Can you work these out from the drawing? Everything is in mm from the part's minimum corner. A direction names the side the tool comes from. Coordinates: 2 decimals unless noted, no trailing zeros. Order: outer loops, then holes, each group sorted by start corner. A loop starts at its lowest first (then second) coordinate and runs counter-clockwise, first axis right, second up. Notation, with made-up numbers: (82.25, 18) - (108.25, 18) arc R27 ccw to (108.25, 43) - close; hole circle Ø3 at (37, -8.5). An arc over 180 degrees is marked (long way). Use CSV: the item, a comma, the result in double quotes. Start each with the question number.
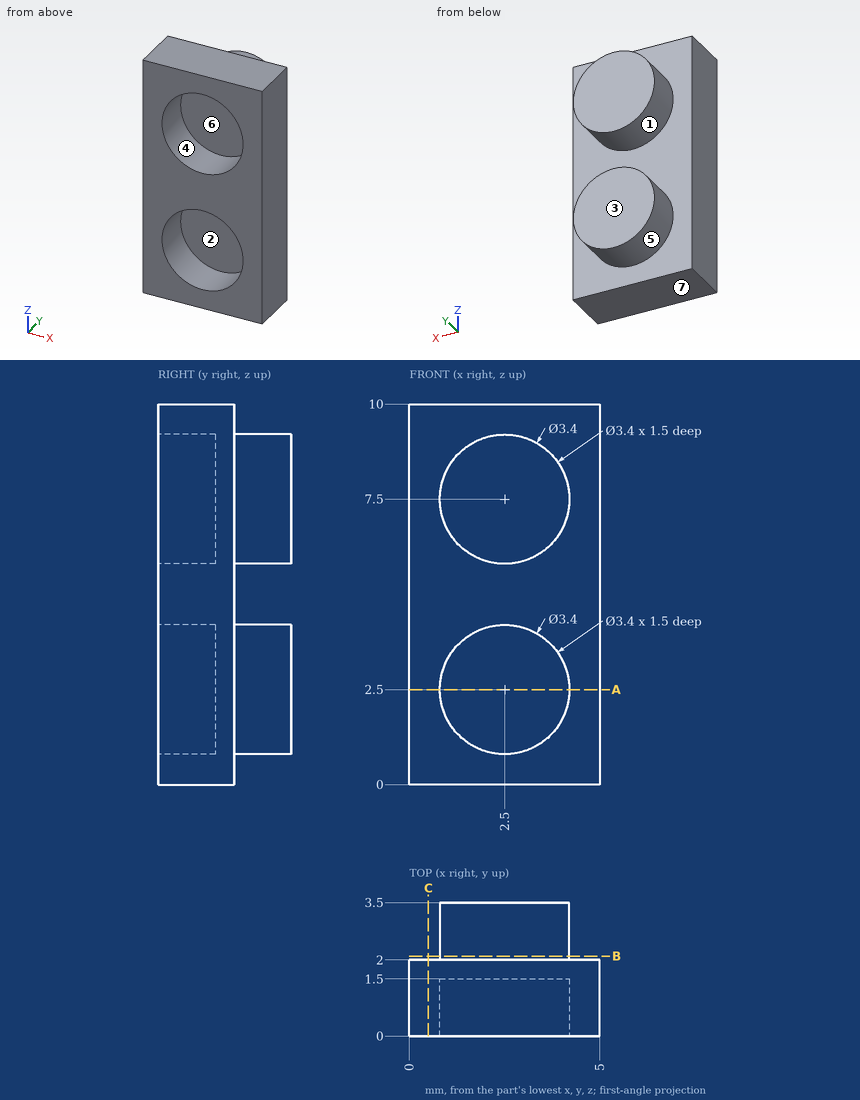
Item 1: Suppose I cut it at C-C on x = 0.5. Write out the boundary of the cut face in (y, z).
Item 2: We'd pull the mould along X, two halves only. Please class the marked faces 4, 5, 6 and 7: released by +X, released by -X, zero draft, split by the parting line, or undercut.
Item 3: Suppose I cut it at A-A on z = 2.5. Write out the boundary of the cut face in (x, y).
Item 4: For pin 1 Ø2.5 at (x, z) = (2.5, 2.5) entering from -Y, with a flat end and sliding along its axis, tell me the tip position at first contact or that it passes through.
Item 5: Please list where these lines run through material, in increasing order: line 1 along Z through (x, y) = (2.5, 0.7); line 2 along Z through (x, y) = (3.75, 0.5); line 3 along Y through (x, z) = (1.25, 6.5). Write a range as from..to.
Item 6: Suppose I cut it at B-B on y = 2.1. Write out the boundary of the cut face in (x, z), then the cut area to 3 significant figures.
Item 7: For the marked faces 1, 2 and 3, which set-ups out of +Z, -Z, +X, -X, +Y, -Y let a thin tool reach every point of the face, with its end or its side?
Here are the results:
1,outline,"(0, 0) - (2, 0) - (2, 10) - (0, 10) - close"
2,face 4,"undercut"
2,face 5,"split by the parting line"
2,face 6,"undercut"
2,face 7,"zero draft"
3,outline,"(0, 0) - (0.8, 0) - (0.8, 1.5) - (4.2, 1.5) - (4.2, 0) - (5, 0) - (5, 2) - (4.2, 2) - (4.2, 3.5) - (0.8, 3.5) - (0.8, 2) - (0, 2) - close"
4,pin 1,"y = 1.5"
5,line 1,"0..0.8, 4.2..5.8, 9.2..10"
5,line 2,"0..1.35, 3.65..6.35, 8.65..10"
5,line 3,"1.5..3.5"
6,outline,"circle Ø3.4 at (2.5, 2.5); circle Ø3.4 at (2.5, 7.5)"
6,area,"18.2 mm^2"
7,face 1,"+Y"
7,face 2,"-Y"
7,face 3,"+Z, -Z, +X, -X, +Y"
